Design review of the part built by this model. Coordinates are the model's own, in mm. A direction names the side the tool comes from. Give positions to 0.01 mm unless a question says otherwise; leave off trailing zeros. Write each loop counter-clockwise with the first axis right and the second up, starting at its lowest first coordinate (ties: lowest second). Pieces come first, ordered by that corner, then holes. Notation, with made-up numbers: (-11.75, -36) -> (45.25, -36) arc R17 cw to (45.25, -4) -> close; hole circle Ø3 at (81.5, 18.25). An arc over 180 degrees is marked (long way). Answer as a JSON object with one key per item and string values.
```python
from build123d import *

# Parameters (mm, degrees)
SKETCH_1_W                  = 84
SKETCH_1_H                  = 80
SKETCH_1_R                  = 14
EXTRUDE_1_DEPTH             = 3
HOLE_WIZARD_M4_1_AT_2_COUNT = 2
HOLE_WIZARD_M4_1_AT_2_PITCH = 50
HOLE_WIZARD_1_D             = 4.5
HOLE_WIZARD_1_DEPTH         = 10
HOLE_WIZARD_1_CSINK_D       = 8.6
HOLE_WIZARD_1_CSINK_ANGLE   = 90
HOLE_WIZARD_1_TIP           = 1.351936393


with BuildPart() as part:
    # 草图1 → 凸台-拉伸1 (new, symmetric)
    with BuildSketch(Plane.XY):
        Rectangle(SKETCH_1_W, SKETCH_1_H)
        Circle(SKETCH_1_R, mode=Mode.SUBTRACT)
    extrude(amount=EXTRUDE_1_DEPTH, both=True)

    # 草图4 → M4 螺纹孔1 (revolve, cut)
    with BuildSketch(Plane(origin=(-42, 25, 0), x_dir=(0, 0, 1), z_dir=(0, 1, 0))):
        Polygon((0, 0), (0, 12.491420021), (1.65, 11.5), (1.65, 0), align=None)
    hole_wizard_m4_1 = revolve(axis=Axis((-48.35, 25, 0), (1, 0, 0)), mode=Mode.SUBTRACT)

    # M4 螺纹孔1 at 2: M4 螺纹孔1 ×2
    with Locations(*[(0, -i * HOLE_WIZARD_M4_1_AT_2_PITCH, 0) for i in range(1, HOLE_WIZARD_M4_1_AT_2_COUNT)]):
        add(hole_wizard_m4_1, mode=Mode.SUBTRACT)

    # 镜向1: M4 螺纹孔1 across plane
    add(hole_wizard_m4_1.mirror(Plane(origin=(0, 0, 0), x_dir=(0, 0, 1), z_dir=(1, 0, 0))), mode=Mode.SUBTRACT)

    # 镜向1 copy 1 sketch → 镜向1 copy 1 (revolve, cut)
    with BuildSketch(Plane(origin=(42, -25, 0), x_dir=(0, 0, 1), z_dir=(0, 1, 0))):
        Polygon((0, 0), (0, -12.491420021), (1.65, -11.5), (1.65, 0), align=None)
    revolve(axis=Axis((48.35, -25, 0), (1, 0, 0)), mode=Mode.SUBTRACT)

    # 打孔尺寸(%根据十字)槽沉头木螺钉的类型1
    with Locations(Plane(origin=(0, 0, 3), x_dir=(-1, 0, 0), z_dir=(0, 0, 1))):
        with Locations((6, 34), (-6, 34)):
            CounterSinkHole(HOLE_WIZARD_1_D / 2, HOLE_WIZARD_1_CSINK_D / 2, depth=HOLE_WIZARD_1_DEPTH, counter_sink_angle=HOLE_WIZARD_1_CSINK_ANGLE)
            with Locations((0, 0, -(HOLE_WIZARD_1_DEPTH + HOLE_WIZARD_1_TIP / 2))):  # 118° drill point
                Cone(0, HOLE_WIZARD_1_D / 2, HOLE_WIZARD_1_TIP, mode=Mode.SUBTRACT)


solid = part.part
```
(1) Clearance check with flat-ended pins moving along their axes: pin 1 (4 mm diameter, centred on x = 6, y = -34, fed in from +Z); pin 2 (2.5 mm diameter, centred on y = 25, z = 0, fed in from +X). State where each tip first meets the part, or that it passes through.
Here are the results:
{"pin 1": "passes through", "pin 2": "stops at x = 30.26"}
(2) The part is to be moulded in two halves that separate along Z. For faces 4 (the cylindrical face through (-36.33, 23.364, -0.215)), 5 (the flat face through (-1, 18, 3)), 6 (the flat face through (-1, 18, -3)), 7 (the flat face through (-1, 40, 0)), say which applies: +Z half, -Z half, draft (parallel to the pull), parting line (faces both ways), or undercut.
Here are the results:
{"face 4": "undercut", "face 5": "+Z half", "face 6": "-Z half", "face 7": "draft"}
(3) We need section B-B, the plane y = -34. State the section outline as (x, z) points, then the cut area to 3 significant figures.
Here are the results:
{"outline": "(-42, -3) -> (-8.25, -3) -> (-8.25, 0.95) -> (-10.3, 3) -> (-42, 3) -> close; (-3.75, -3) -> (3.75, -3) -> (3.75, 0.95) -> (1.7, 3) -> (-1.7, 3) -> (-3.75, 0.95) -> close; (8.25, -3) -> (42, -3) -> (42, 3) -> (10.3, 3) -> (8.25, 0.95) -> close", "area": "442 mm²"}
(4) We need section A-A, the plane x = 0. State the section outline as (y, z) points, then the cut area to 3 significant figures.
Here are the results:
{"outline": "(-40, -3) -> (-14, -3) -> (-14, 3) -> (-40, 3) -> close; (14, -3) -> (40, -3) -> (40, 3) -> (14, 3) -> close", "area": "312 mm²"}
(5) For line 1 along Y through (x, z) = (-33.25, 0); line 2 along Y through (x, z) = (-32.5, 0.9); line 3 along Z through (x, y) = (-36, 25), list the stretches that pass through material, from the lowest coordinate up.
Here are the results:
{"line 1": "y = -40 to -26.65, -23.35 to 23.35, 26.65 to 40", "line 2": "y = -40 to -26.38, -23.62 to 23.62, 26.38 to 40", "line 3": "z = -3 to -1.65, 1.65 to 3"}
(6) We need section C-C, the plane y = -7. State the section outline as (x, z) points, then the cut area to 3 significant figures.
Here are the results:
{"outline": "(-42, -3) -> (-12.12, -3) -> (-12.12, 3) -> (-42, 3) -> close; (12.12, -3) -> (42, -3) -> (42, 3) -> (12.12, 3) -> close", "area": "359 mm²"}
(7) For faces 1 (the flat face through (-42, -1, 0)), 2 (the cylindrical face through (-36.33, -26.636, -0.215)), 3 (the cylindrical face through (36.33, -26.636, -0.215)), list the 3-axis set-ups (+Z, -Z, +X, -X, +Y, -Y) from which the entire face can be reached by the end or side of a thin tool; tool diameter is ignored.
Here are the results:
{"face 1": "+Z, -Z, -X, +Y, -Y", "face 2": "-X", "face 3": "+X"}
